```python
from build123d import *

# Parameters (mm, degrees)
MODEL_W                    = 142.95
MODEL_H                    = 122.297505408
MODEL_W_2                  = 14
MODEL_H_2                  = 14
SALIENTE_EXTRUIR1_DEPTH    = 0.75
CROQUIS2_W                 = 15
CROQUIS2_H                 = 30
CORTAR_EXTRUIR1_DEPTH      = 183.563364442
CROQUIS3_W                 = 17
CROQUIS3_H                 = 17
SALIENTE_EXTRUIR2_DEPTH    = 1.5
S_LIDO_MOVER_COPIAR1_ANGLE = 180


with BuildPart() as part:
    # Model → Saliente-Extruir1 (new, symmetric)
    with BuildSketch(Plane.XY):
        with Locations((67.525, 57.198752704)):
            Rectangle(MODEL_W, MODEL_H)
        with Locations((58, 42)):
            Rectangle(MODEL_W_2, MODEL_H_2, mode=Mode.SUBTRACT)
        Polygon((18.593146641, 87.427779239), (29.317768845, 78.428752704), (38.316795381, 89.153374907), (27.592173177, 98.152401443), align=None, mode=Mode.SUBTRACT)
        Polygon((103.814404332, 23.723648739), (114.539026536, 14.724622204), (105.54, 4), (94.815377796, 12.999026536), align=None, mode=Mode.SUBTRACT)
        Polygon((33.186293283, 75.182675275), (43.910915486, 66.183648739), (52.909942022, 76.908270943), (42.185319818, 85.907297479), align=None, mode=Mode.SUBTRACT)
        Polygon((20.510973464, 14.724622204), (29.51, 4), (40.234622204, 12.999026536), (31.235595668, 23.723648739), align=None, mode=Mode.SUBTRACT)
        with Locations((77.05, 42)):
            Rectangle(MODEL_W_2, MODEL_H_2, mode=Mode.SUBTRACT)
        Polygon((92.864680182, 85.907297479), (101.863706717, 75.182675275), (91.139084514, 66.183648739), (82.140057978, 76.908270943), align=None, mode=Mode.SUBTRACT)
        Polygon((107.457826823, 98.152401443), (116.456853359, 87.427779239), (105.732231155, 78.428752704), (96.733204619, 89.153374907), align=None, mode=Mode.SUBTRACT)
        Polygon((4, 99.672883204), (14.724622204, 90.673856668), (23.723648739, 101.398478872), (12.999026536, 110.397505408), align=None, mode=Mode.SUBTRACT)
        Polygon((120.325377796, 90.673856668), (111.326351261, 101.398478872), (122.050973464, 110.397505408), (131.05, 99.672883204), align=None, mode=Mode.SUBTRACT)
    extrude(amount=SALIENTE_EXTRUIR1_DEPTH, both=True)

    # Croquis2 → Cortar-Extruir1 (cut, through all)
    with BuildSketch(Plane.XY.offset(0.75)):
        with Locations((67.525, 118.347505408)):
            Rectangle(CROQUIS2_W, CROQUIS2_H)
    extrude(amount=-CORTAR_EXTRUIR1_DEPTH, mode=Mode.SUBTRACT)

    # Croquis3 → Saliente-Extruir2 (add)
    with BuildSketch(Plane(origin=(0, 0, -0.75), x_dir=(-1, 0, 0), z_dir=(0, 0, -1))):
        Polygon((-57.925, 101.247505408), (-77.125, 101.247505408), (-77.125, 116.247505408), (-136.9, 116.247505408), (-136.9, -1.85), (1.85, -1.85), (1.85, 116.247505408), (-57.925, 116.247505408), align=None)
        Polygon((-29.32511475, 1.886751921), (-18.397725385, 14.909507454), (-31.420480918, 25.836896818), (-42.347870283, 12.814141285), align=None, mode=Mode.SUBTRACT)
        with Locations((-58, 42)):
            Rectangle(CROQUIS3_W, CROQUIS3_H, mode=Mode.SUBTRACT)
        with Locations((-77.05, 42)):
            Rectangle(CROQUIS3_W, CROQUIS3_H, mode=Mode.SUBTRACT)
        Polygon((-105.72488525, 1.886751921), (-92.702129717, 12.814141285), (-103.629519082, 25.836896818), (-116.652274615, 14.909507454), align=None, mode=Mode.SUBTRACT)
        Polygon((-1.886751921, 99.487997954), (-12.814141285, 112.510753487), (-25.836896818, 101.583364122), (-14.909507454, 88.560608589), align=None, mode=Mode.SUBTRACT)
        Polygon((-16.479898562, 87.242893989), (-27.407287927, 100.265649522), (-40.43004346, 89.338260158), (-29.502654095, 76.315504625), align=None, mode=Mode.SUBTRACT)
        Polygon((-31.073045204, 74.997790025), (-42.000434568, 88.020545558), (-55.023190101, 77.093156193), (-44.095800737, 64.07040066), align=None, mode=Mode.SUBTRACT)
        Polygon((-90.954199263, 64.07040066), (-80.026809899, 77.093156193), (-93.049565432, 88.020545558), (-103.976954796, 74.997790025), align=None, mode=Mode.SUBTRACT)
        Polygon((-105.547345905, 76.315504625), (-94.61995654, 89.338260158), (-107.642712073, 100.265649522), (-118.570101438, 87.242893989), align=None, mode=Mode.SUBTRACT)
        Polygon((-120.140492546, 88.560608589), (-109.213103182, 101.583364122), (-122.235858715, 112.510753487), (-133.163248079, 99.487997954), align=None, mode=Mode.SUBTRACT)
    extrude(amount=SALIENTE_EXTRUIR2_DEPTH)


with BuildPart() as part_1:
    # Sólido-Mover/Copiar1: moved
    add(part.part.rotate(Axis((0, 57.198752704, -0.75), (1, 0, 0)), S_LIDO_MOVER_COPIAR1_ANGLE))


solid = part_1.part
```
CAD build for the part. Positions are in the model's coordinates, mm. A direction names the side the tool comes from. Round coordinates to 2 decimals unless told otherwise and drop trailing zeros. Write each loop counter-clockwise with the first axis right and the second up, starting at its lowest first coordinate (ties: lowest second). Pieces come first, ordered by that corner, then holes.
Item 1: Tool access for faces 1 (the flat face through (102.02, 20.81, -1.51)), 2 (the flat face through (97.557, 44.787, -0.01)): list every direction of +Z, -Z, +X, -X, +Y, -Y with a clear straight run to the whole face (end or side of a thin tool).
Filled in:
face 1: +Z, -Z
face 2: +Z
Item 2: Band-saw the part on A-A on y = 76. Write the cut outline in (x, z).
Filled in:
outline: (-3.95, -2.25) - (51, -2.25) - (51, -0.75) - (49.5, -0.75) - (49.5, 0.75) - (-1.85, 0.75) - (-1.85, -0.75) - (-3.95, -0.75) - close; (65, -2.25) - (70.05, -2.25) - (70.05, -0.75) - (68.55, -0.75) - (68.55, 0.75) - (66.5, 0.75) - (66.5, -0.75) - (65, -0.75) - close; (84.05, -2.25) - (139, -2.25) - (139, -0.75) - (136.9, -0.75) - (136.9, 0.75) - (85.55, 0.75) - (85.55, -0.75) - (84.05, -0.75) - close
Item 3: Band-saw the part on D-D on y = 93. Write the cut outline in (x, z).
Filled in:
outline: (-3.95, -2.25) - (28.46, -2.25) - (28.46, -0.75) - (26.13, -0.75) - (26.13, 0.75) - (-1.85, 0.75) - (-1.85, -0.75) - (-3.95, -0.75) - close; (33.19, -2.25) - (101.86, -2.25) - (101.86, -0.75) - (99.9, -0.75) - (99.9, 0.75) - (35.15, 0.75) - (35.15, -0.75) - (33.19, -0.75) - close; (106.59, -2.25) - (139, -2.25) - (139, -0.75) - (136.9, -0.75) - (136.9, 0.75) - (108.92, 0.75) - (108.92, -0.75) - (106.59, -0.75) - close
Item 4: Drop flat-ended pins along their axis: pin 1 Ø1.2 at (y, z) = (68, 0) entering from +X; pin 2 Ø1.6 at (x, z) = (61, 0) entering from -Y; pin 3 Ø1.7 at (y, z) = (72, 0) entering from +X; pin 4 Ø7 at (x, y) = (26.5, 22.5) entering from +Z. Give the stop position or say it passes through.
Filled in:
pin 1: stops at x = 136.9
pin 2: stops at y = 11.05
pin 3: stops at x = 139
pin 4: stops at z = -0.75
Item 5: Band-saw the part on B-B on x = 100. Give the number of separate pieces and of enclosed holes in the cut face, then the cut area to 3 significant figures.
Filled in:
separate pieces: 4
enclosed holes: 0
area: 278 mm2
Item 6: Drill centre lines: L1, parallel to X at y = 69, z = 0.1; L2, parallel to X at y = 67.5, z = -1.8; L3, parallel to Y at x = 62, z = -1.2. Where is each one in solid material? Low to high.
Filled in:
L1: x = -1.85 to 49.5, 66.5 to 68.55, 85.55 to 136.9
L2: x = -3.95 to 51, 65 to 70.05, 84.05 to 139
L3: y = 11.05 to 65.4, 79.4 to 118.35
